Part model, mm, in its own coordinate system. Face numbers are marked on the shaded views. Give positions to 0.01 mm unless a question says otherwise; leave off trailing zeros. Write each loop counter-clockwise with the first axis right and the second up, starting at its lowest first coordinate (ties: lowest second). Pieces come first, ordered by that corner, then holes.
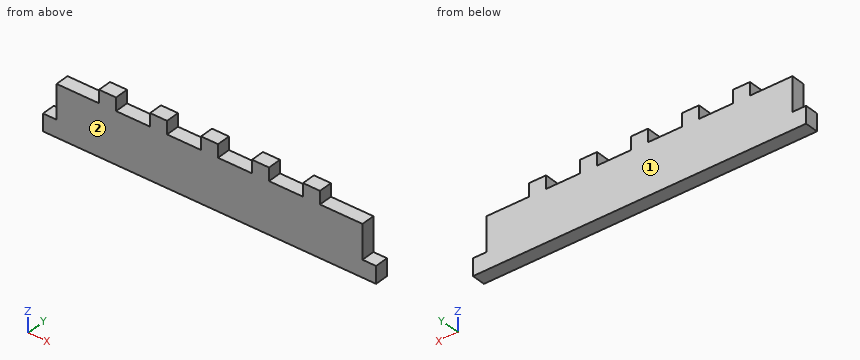
```python
from build123d import *

# Parameters (mm, degrees)
BOSS_EXTRUDE1_DEPTH = 5.08
SKETCH2_W           = 6.35
SKETCH2_H           = 5.08
BOSS_EXTRUDE2_DEPTH = 4.826
LPATTERN1_COUNT     = 5
LPATTERN1_PITCH     = 19.05


with BuildPart() as part:
    # Sketch1 → Boss-Extrude1 (new body)
    with BuildSketch(Plane(origin=(0, 0, 0), x_dir=(1, 0, 0), z_dir=(0, 1, 0))):
        Polygon((0, 0), (114.3, 0), (114.3, 12.7), (119.38, 12.7), (119.38, 19.05), (114.3, 19.05), (0, 19.05), (-5.08, 19.05), (-5.08, 12.7), (0, 12.7), align=None)
    extrude(amount=BOSS_EXTRUDE1_DEPTH)

    # Sketch2 → Boss-Extrude2 (add)
    with BuildSketch(Plane.XY):
        with Locations((19.05, 2.54)):
            Rectangle(SKETCH2_W, SKETCH2_H)
    boss_extrude2 = extrude(amount=BOSS_EXTRUDE2_DEPTH)

    # LPattern1: Boss-Extrude2 ×5
    with Locations(*[(i * LPATTERN1_PITCH, 0, 0) for i in range(1, LPATTERN1_COUNT)]):
        add(boss_extrude2)


solid = part.part
```
1) Pin check, flat tips, straight feed: pin 1 Ø1.5 at (y, z) = (3.5, -5.5) entering from +X; pin 2 Ø1.5 at (x, y) = (46, 3) entering from +Z; pin 3 Ø2.5 at (y, z) = (2.5, 1) entering from -X. Stop position of each tip, or through.
Answers follow:
pin 1: stops at x = 114.3
pin 2: stops at z = 0
pin 3: stops at x = 0
2) Saw through at C-C, the plane x = 106.5. Write the cut outline in (y, z).
Answers follow:
outline: (0, -19.05) - (5.08, -19.05) - (5.08, 0) - (0, 0) - close
3) Saw through at B-B, the plane z = -6.25. Write the cut outline in (x, y).
Answers follow:
outline: (0, 0) - (114.3, 0) - (114.3, 5.08) - (0, 5.08) - close
4) Saw through at A-A, the plane y = 2.6. Write the cut outline in (x, z) (3 decimals).
Answers follow:
outline: (-5.08, -19.05) - (119.38, -19.05) - (119.38, -12.7) - (114.3, -12.7) - (114.3, 0) - (98.425, 0) - (98.425, 4.826) - (92.075, 4.826) - (92.075, 0) - (79.375, 0) - (79.375, 4.826) - (73.025, 4.826) - (73.025, 0) - (60.325, 0) - (60.325, 4.826) - (53.975, 4.826) - (53.975, 0) - (41.275, 0) - (41.275, 4.826) - (34.925, 4.826) - (34.925, 0) - (22.225, 0) - (22.225, 4.826) - (15.875, 4.826) - (15.875, 0) - (0, 0) - (0, -12.7) - (-5.08, -12.7) - close
5) Wall check: L1, parallel to X at y = 1.75, z = 2 (3 decimals); L2, parallel to Z at x = 85, y = 4.15; L3, parallel to X at y = 2.8, z = -1. Give the ranges that are in metal, low to high.
Answers follow:
L1: x = 15.875 to 22.225, 34.925 to 41.275, 53.975 to 60.325, 73.025 to 79.375, 92.075 to 98.425
L2: z = -19.05 to 0
L3: x = 0 to 114.3
6) Two-plate mould, pull along Y, no slides. Class the marked faces 1 and 2: +Y half, -Y half, draft (parallel to the pull), parting line (faces both ways), or undercut.
Answers follow:
face 1: +Y half
face 2: -Y half
